The listing builds one solid part. Answer for the finished solid, in the listing's coordinates (mm). A direction names the side the tool comes from. Round coordinates to 2 decimals unless told otherwise and drop trailing zeros. Write each loop counter-clockwise with the first axis right and the second up, starting at its lowest first coordinate (ties: lowest second). Pieces come first, ordered by that corner, then holes. Notation, with made-up numbers: M 23,-28 L 30,-28 A10 ccw 30,-13 Z; hole C 7,-1.75 d5. An arc over 180 degrees is marked long. One line per item, written item: value. Start each with the question number.
(1) Section A-A (x = 0) is taken. Determine the outline of the cut face in (y, z).
(2) Consider probe 1 along Y at (x, z) = (10, -9); probe 2 along Z at (x, y) = (-6, 160); probe 3 along Y at (x, z) = (-21, 11.5). Determine where each line is inside the solid, lowest interval first.
(3) Section C-C (z = -2.5) is taken. Determine the outline of the cut face in (x, y), plus the area to 3 significant figures.
(4) Section D-D (y = 0) is taken. Determine the outline of the cut face in (x, z).
(5) For a pull along X with two mould halves and no side action, classify faces 5 (the flat face through (29.236, 102.94, 0.14)), 6 (the flat face through (-44.545, 79.015, -0.14)), 7 (the flat face through (0, 65, -10)) as released by +X, released by -X, zero draft, split by the parting line, or undercut.
(6) For faces 1 (the flat face through (-40, 153, 4)), 2 (the cylindrical face through (0.56, 166.93, -2.87)), 3 (the flat face through (40, 153, 4)), 4 (the cylindrical face through (0, 70, 0)), determine the directions among +Z, -Z, +X, -X, +Y, -Y from which every point of the face is accessible in a straight line to the end or side of a thin tool.
(7) Given P1, Ø3, axis at x = 46, y = 78.5, coming from the -Z side; P2, Ø4, axis at y = -26, z = -2, coming from the -X side; P3, Ø9, axis at y = 156.5, z = -7, coming from the +X side, each flat-ended and moving along its own axis, determine where each tip first touches the part or whether it passes through.
(8) Section B-B (y = 160) is taken. Determine the outline of the cut face in (x, z).
Autodesk Inventor part; units mm, degrees
ref_plane "Arbeitsebene1" through (0, 0, 0) normal (1, 0, 0) x (0, 1, 0)
ref_plane "XZ Plane" through (0, 0, 0) normal (0, 1, 0) x (-1, 0, 0)
ref_plane "XY Plane" through (0, 0, 0) normal (0, 0, 1) x (1, 0, 0)
sketch "Skizze1" plane through (0, 0, 0) normal (0, 0, 1) x (1, 0, 0)
  circle A0 centre (0, 0) radius 60
  line L0 (-58.6889, 12.4747) -> (-30, 147.4452)
  line L1 (58.6889, 12.4747) -> (30, 147.4452)
  line L2 (30, 147.4452) -> (-30, 147.4452)
  line L3 (0, 0) -> (0, 147.4452) construction
  dimension "d0" = 120
  dimension "d1" = 24
  dimension "d2" = 60
extrude "Extrusion1" add sketch "Skizze1" along normal mid plane 30 contours A0
extrude "Extrusion2" add sketch "Skizze1" along normal mid plane 20 contours A0 L0 L2 L1
sketch "Skizze2" plane through (0, 0, 15) normal (0, 0, 1) x (1, 0, 0)
  circle A0 centre (0, 0) radius 50
  dimension "d7" = 100
extrude "Extrusion3" cut sketch "Skizze2" against normal up to surface (30 mm away)
ref_plane "Arbeitsebene1" through (0, 0, 0) normal (1, 0, 0) x (0, 1, 0)
sketch "Skizze3" plane through (0, 0, 0) normal (1, 0, 0) x (0, 1, 0)
  line L0 (147.4452, 10) -> (12.4747, 10)
  line L1 (12.4747, 10) -> (12.4747, 10)
  line L2 (12.4747, 10) -> (147.4452, 10)
  circle A0 centre (160, 0) radius 15
  circle A1 centre (160, 0) radius 7.5
  point P0 (0, 0)
  dimension "d11" = 30
  dimension "d12" = 160
  dimension "d13" = 15
extrude "Extrusion4" add sketch "Skizze3" along normal mid plane 80
sketch "Skizze4" plane through (0, 0, 10) normal (0, 0, 1) x (1, 0, 0)
  line L0 (-21.9022, 137.4452) -> (21.9022, 137.4452)
  line L1 (21.9022, 137.4452) -> (38.7218, 58.3148)
  line L2 (-38.7218, 58.3148) -> (-21.9022, 137.4452)
  line L3 (0, 0) -> (0, 147.2716) construction
  line L4 (-30, 147.4452) -> (-58.6889, 12.4747)
  line L5 (58.6889, 12.4747) -> (30, 147.4452)
  line L6 (30, 147.4452) -> (-30, 147.4452)
  arc A0 (38.7218, 58.3148) -> (-38.7218, 58.3148) centre (0, 0) ccw
  circle A1 centre (0, 0) radius 60
  dimension "d16" = 10
  dimension "d17" = 10
  dimension "d18" = 70
extrude "Extrusion5" cut sketch "Skizze4" against normal up to surface (20 mm away) contours L0 L1 A0 L2
fillet "Rundung1" radius 5 2 edges at (-38.7218, 58.3148, 0) (38.7218, 58.3148, 0)
fillet "Rundung2" radius 2 2 edges at (21.9022, 137.4452, 0) (-21.9022, 137.4452, 0)
properties part number "Excercise4" material "Stahl, galvanisiert"
Recorded:
1. outline: M -60,-15 L -50,-15 L -50,15 L -60,15 Z; M 50,-15 L 60,-15 L 60,-10 L 70,-10 L 70,10 L 60,10 L 60,15 L 50,15 Z; M 137.45,-10 L 147.45,-10 L 147.45,-8.21 A15 ccw long 147.45,8.21 L 147.45,10 L 137.45,10 Z; hole C 160,0 d15
2. probe 1: y = -59.16 to -48.99, 48.99 to 69.28, 137.45 to 147.45, 148 to 172
2. probe 2: z = -15 to -7.5, 7.5 to 15
2. probe 3: y = -56.2 to -45.38, 45.38 to 56.2, 150.37 to 169.63
3. outline: M -58.69,12.47 A60 ccw long 58.69,12.47 L 30.48,145.21 L 40,145.21 L 40,152.93 L -40,152.93 L -40,145.21 L -30.48,145.21 Z; M -40,167.07 L 40,167.07 L 40,174.79 L -40,174.79 Z; hole C 0,0 d100; hole M -36.43,69.08 A5 ccw -29.44,63.51 A70 cw 29.44,63.51 A5 ccw 36.43,69.08 L 22.24,135.86 A2 ccw 20.28,137.45 L -20.28,137.45 A2 ccw -22.24,135.86 Z
3. area: 8,230 mm2
4. outline: M -60,-15 L -50,-15 L -50,15 L -60,15 Z; M 50,-15 L 60,-15 L 60,15 L 50,15 Z
5. face 5: undercut
5. face 6: released by -X
5. face 7: zero draft
6. face 1: +Z, -Z, -X, +Y
6. face 2: +X, -X
6. face 3: +Z, -Z, +X, +Y
6. face 4: +Z, -Z
7. P1: stops at z = -10
7. P2: stops at x = -54.99
7. P3: stops at x = 40
8. outline: M -40,-15 L 40,-15 L 40,-7.5 L -40,-7.5 Z; M -40,7.5 L 40,7.5 L 40,15 L -40,15 Z
